```python
from build123d import *

# Parameters (mm, degrees)
SKETCH_R           = 50
PAD_DEPTH          = 10
SKETCH001_R        = 5
POCKET_DEPTH       = 5
POLARPATTERN_COUNT = 10
SKETCH002_W        = 40
SKETCH002_H        = 40
PAD001_DEPTH       = 10
SKETCH004_R        = 4.452809


with BuildPart() as part:
    # Sketch → Pad (new body)
    with BuildSketch(Plane.XY):
        Circle(SKETCH_R)
    extrude(amount=PAD_DEPTH)

    # Sketch001 (on Face3 of Pad) → Pocket (cut)
    with BuildSketch(Plane.XY.offset(10)):
        with Locations((0, 40)):
            Circle(SKETCH001_R)
    pocket = extrude(amount=-POCKET_DEPTH, mode=Mode.SUBTRACT)

    # PolarPattern: Pocket ×10 about axis
    polarpattern_axis = Axis((0, 0, 0), (0, 0, 1))
    for i in range(1, POLARPATTERN_COUNT):
        add(pocket.rotate(polarpattern_axis, i * 360 / POLARPATTERN_COUNT), mode=Mode.SUBTRACT)

    # Sketch002 (on Face3 of PolarPattern) → Pad001 (join)
    with BuildSketch(Plane.XY.offset(10)):
        Rectangle(SKETCH002_W, SKETCH002_H)
    extrude(amount=PAD001_DEPTH)

    # Sketch003 → Revolution (revolve)
    with BuildSketch(Plane.XZ):
        with BuildLine():
            ThreePointArc((0, 10), (25, 35), (0, 60))
            Line((0, 60), (0, 10))
        make_face()
    revolve(axis=Axis((0, 0, 0), (0, 0, 1)))

    # Sketch004 → Groove (revolve, cut)
    with BuildSketch(Plane.XZ):
        with Locations((7.491299, 58.851215)):
            Circle(SKETCH004_R)
    revolve(axis=Axis((0, 0, 0), (0, 0, 1)), mode=Mode.SUBTRACT)


solid = part.part
```
Verification items for the finished model (mm, model axes). A direction names the side the tool comes from. Round coordinates to 2 decimals unless told otherwise and drop trailing zeros. Write each loop counter-clockwise with the first axis right and the second up, starting at its lowest first coordinate (ties: lowest second). Pieces come first, ordered by that corner, then holes.
1. Section check D-D on x = 31. Enter the section's corners in (y, z), plus the area to 3 significant figures.
2. Section check A-A on x = -22.5. Enter the section's corners in (y, z).
3. Scan lines: L1, parallel to Y at x = 0.5, z = 5.5; L2, parallel to X at y = 0, z = 34; L3, parallel to X at y = -15, z = 27.5. Record each from-to range of solid material in increasing order.
4. Access from +Z, -Z, +X, -X, +Y, -Y to the whole of each face (thin tool, end or side, straight path). Record for faces 1 (the cylindrical face through (41.22, -16.22, 7.54)), 2 (the flat face through (22, 1, 10)), 3 (the flat face through (0, -20, 15)).
5. Draft check along X on faces 4 (the flat face through (20, 0, 15)), 5 (the cylindrical face through (-18.65, 33.53, 7.54)), 6 (the cylindrical face through (0.651, -44.957, 7.535)), 7 (the flat face through (0, 20, 15)). Enter one of: +X half, -X half, draft (parallel to the pull), parting line (faces both ways), or undercut.
6. Gauge pin test, flat ends, axial feed: P1, Ø6, axis at x = -10.5, y = 7, coming from the +Z side; P2, Ø11, axis at x = 0.5, y = -40, coming from the +Z side; P3, Ø8, axis at y = -9, z = 13, coming from the +X side; P4, Ø13, axis at x = 38.04, y = -12.36, coming from the -Z side. Record the tip position at first contact, or that the pin passes through.
7. Section check B-B on y = 21.5. Enter the section's corners in (x, z), plus the area to 3 significant figures.
8. Section check C-C on y = -40. Enter the section's corners in (x, z).
Answer:
1. outline: (-39.23, 0) - (39.23, 0) - (39.23, 10) - (-39.23, 10) - close
1. area: 785 mm2
2. outline: (-44.65, 0) - (44.65, 0) - (44.65, 10) - (37.26, 10) - (37.26, 5) - (27.46, 5) - (27.46, 10) - (-27.46, 10) - (-27.46, 5) - (-37.26, 5) - (-37.26, 10) - (-44.65, 10) - close; circle Ø21.79 at (0, 35)
3. L1: y = -50 to -44.97, -35.03 to 35.03, 44.97 to 50
3. L2: x = -24.98 to 24.98
3. L3: x = -18.54 to 18.54
4. face 1: +Z
4. face 2: none
4. face 3: +X, -X, -Y
5. face 4: +X half
5. face 5: undercut
5. face 6: undercut
5. face 7: draft
6. P1: stops at z = 57.14
6. P2: stops at z = 10
6. P3: stops at x = 49.59
6. P4: stops at z = 0
7. outline: (-45.14, 0) - (45.14, 0) - (45.14, 10) - (-45.14, 10) - close; circle Ø25.51 at (0, 35)
7. area: 1,410 mm2
8. outline: (-30, 0) - (30, 0) - (30, 10) - (5, 10) - (5, 5) - (-5, 5) - (-5, 10) - (-30, 10) - close
